CAD build for the part. Positions are in the model's coordinates, mm. Face numbers are marked on the shaded views. Round coordinates to 2 decimals unless told otherwise and drop trailing zeros. Write each loop counter-clockwise with the first axis right and the second up, starting at its lowest first coordinate (ties: lowest second). Pieces come first, ordered by that corner, then holes. Notation, with made-up numbers: (-32, 30) - (9, 30) arc R20 ccw to (9, 40) - close; hole circle Ø5 at (56.5, 87.5). An arc over 180 degrees is marked (long way). Put each result on its own line as item: value. Start each with the question number.
Item 1: Cut at B-B (y = 12.7). Give the cut face in (x, z) (3 decimals), and give its area (3 significant figures).
Item 2: Cut at D-D (x = 12.7). Give the cut face in (y, z) (3 decimals), and give its area (3 significant figures).
Item 3: Cut at A-A (x = 1.75). Give the cut face in (y, z) (3 decimals).
Item 4: Cut at C-C (z = -26). Give the cut face in (x, y) (3 decimals).
Item 5: Drill centre lines: line 1 (Z direction, x = 12.7, y = 2.55); line 2 (Y direction, x = 0.8, z = -12.7); line 3 (X direction, y = 15.5, z = -36) (3 decimals). Where is each one in solid material? Low to high. Write a range as from..to.
Item 6: Mould opens along Y. For the marked faces 1, 2 and 3 say: released by +Y, released by -Y, zero draft, split by the parting line, or undercut.
Item 7: Pin check, flat tips, straight feed: pin 1 Ø4 at (y, z) = (18.5, -30) entering from +X (3 decimals); pin 2 Ø10 at (x, z) = (17.5, -34) entering from +Y (3 decimals). Stop position of each tip, or through.
```python
from build123d import *

# Parameters (mm, degrees)
SKETCH1_W               = 25.4
SKETCH1_H               = 50.8
SKETCH1_R               = 3.2639
BOSS_EXTRUDE1_DEPTH     = 3.175
SKETCH2_W               = 3.175
SKETCH2_H               = 50.8
BOSS_EXTRUDE2_DEPTH     = 22.225
SKETCH3_R               = 3.2639
CUT_EXTRUDE1_DEPTH      = 22.225
FILLET2_R               = 2.54
CUT_EXTRUDE3_DEPTH      = 23.225
CUT_EXTRUDE3_DEPTH_BACK = 4.175
FILLET3_R               = 3.175
FILLET4_R               = 3.175


with BuildPart() as part:
    # Sketch1 → Boss-Extrude1 (new body)
    with BuildSketch(Plane(origin=(0, 0, 0), x_dir=(1, 0, 0), z_dir=(0, 1, 0))):
        with Locations((12.7, 25.4)):
            Rectangle(SKETCH1_W, SKETCH1_H)
        with Locations((12.7, 38.1)):
            Circle(SKETCH1_R, mode=Mode.SUBTRACT)
        with Locations((12.7, 12.7)):
            Circle(SKETCH1_R, mode=Mode.SUBTRACT)
    extrude(amount=BOSS_EXTRUDE1_DEPTH)

    # Sketch2 → Boss-Extrude2 (add)
    with BuildSketch(Plane(origin=(0, 3.175, 0), x_dir=(1, 0, 0), z_dir=(0, 1, 0))):
        with Locations((1.5875, 25.4)):
            Rectangle(SKETCH2_W, SKETCH2_H)
    extrude(amount=BOSS_EXTRUDE2_DEPTH)

    # Sketch3 → Cut-Extrude1 (cut)
    with BuildSketch(Plane(origin=(3.175, 0, 0), x_dir=(0, 0, -1), z_dir=(1, 0, 0))):
        with Locations((12.7, 12.7)):
            Circle(SKETCH3_R)
        with Locations((38.1, 12.7)):
            Circle(SKETCH3_R)
    extrude(amount=-CUT_EXTRUDE1_DEPTH, mode=Mode.SUBTRACT)

    # Fillet2
    fillet2_edges = [part.edges().sort_by_distance(p)[0] for p in [
        (3.175, 3.175, -25.4),
    ]]
    fillet(fillet2_edges, radius=FILLET2_R)

    # Sketch4 → Cut-Extrude3 (cut, two sides)
    with BuildSketch(Plane(origin=(0, 3.175, 0), x_dir=(1, 0, 0), z_dir=(0, 1, 0))) as cut_extrude3_sk:
        Polygon((25.4, 0), (25.4, 12.7), (3.175, 0), align=None)
        Polygon((25.4, 50.8), (25.4, 38.1), (3.175, 50.8), align=None)
    extrude(amount=CUT_EXTRUDE3_DEPTH, mode=Mode.SUBTRACT)
    extrude(cut_extrude3_sk.sketch, amount=-CUT_EXTRUDE3_DEPTH_BACK, mode=Mode.SUBTRACT)

    # Fillet3
    fillet3_edges = [part.edges().sort_by_distance(p)[0] for p in [
        (1.5875, 25.4, 0),
    ]]
    fillet(fillet3_edges, radius=FILLET3_R)

    # Fillet4
    fillet4_edges = [part.edges().sort_by_distance(p)[0] for p in [
        (1.5875, 25.4, -50.8),
    ]]
    fillet(fillet4_edges, radius=FILLET4_R)


solid = part.part
```
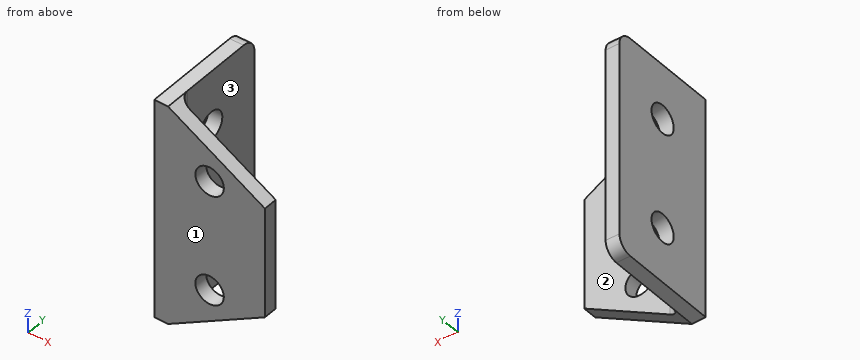
Output values:
1. outline: (0, -50.8) - (3.175, -50.8) - (3.175, -41.364) - (0, -41.364) - close; (0, -34.836) - (3.175, -34.836) - (3.175, -15.964) - (0, -15.964) - close; (0, -9.436) - (3.175, -9.436) - (3.175, 0) - (0, 0) - close
1. area: 120 mm2
2. outline: (0, -45.357) - (3.175, -45.357) - (3.175, -41.364) - (0, -41.364) - close; (0, -34.836) - (3.175, -34.836) - (3.175, -15.964) - (0, -15.964) - close; (0, -9.436) - (3.175, -9.436) - (3.175, -5.443) - (0, -5.443) - close
2. area: 85.3 mm2
3. outline: (0, -50.8) - (22.225, -50.8) arc R3.175 ccw to (25.4, -47.625) - (25.4, -3.175) arc R3.175 ccw to (22.225, 0) - (0, 0) - close; hole circle Ø6.528 at (12.7, -38.1); hole circle Ø6.528 at (12.7, -12.7)
4. outline: (0, 0) - (25.4, 0) - (25.4, 3.175) - (5.715, 3.175) arc R2.54 cw to (3.175, 5.715) - (3.175, 25.4) - (0, 25.4) - close
5. line 1: -45.36..-41.36, -34.84..-15.96, -9.44..-5.44
5. line 2: 0..9.44, 15.96..25.4
5. line 3: 0..3.175
6. face 1: released by -Y
6. face 2: released by +Y
6. face 3: zero draft
7. pin 1: x = 3.175
7. pin 2: y = 3.175
